```python
from build123d import *

# Parameters (mm, degrees)
SKETCH1_W               = 82.8
SKETCH1_H               = 213.8
SKETCH1_R               = 0.8
PCB_EXTRUDE_DEPTH       = 1.6
SKETCH3_R               = 1.5
SOLAR_HOLE_DEPTH        = 1.6
CUT_EXTRUDE1_DEPTH      = 115.647852139
CUT_EXTRUDE1_DEPTH_BACK = 115.647852139
SKETCH8_W               = 82.8
SKETCH8_H               = 114.4
M2_CLEARANCE_HOLE1_D    = 2.6


with BuildPart() as part:
    # Sketch1 → pcb extrude (new body)
    with BuildSketch(Plane.XY):
        Rectangle(SKETCH1_W, SKETCH1_H)
        with Locations((-39.5, -27)):
            Circle(SKETCH1_R, mode=Mode.SUBTRACT)
        with Locations((39.5, -27)):
            Circle(SKETCH1_R, mode=Mode.SUBTRACT)
        with Locations((-39.5, 87)):
            Circle(SKETCH1_R, mode=Mode.SUBTRACT)
        with Locations((-39.5, 57)):
            Circle(SKETCH1_R, mode=Mode.SUBTRACT)
        with Locations((-39.5, 27)):
            Circle(SKETCH1_R, mode=Mode.SUBTRACT)
        with Locations((-39.5, -57)):
            Circle(SKETCH1_R, mode=Mode.SUBTRACT)
        with Locations((-39.5, -87)):
            Circle(SKETCH1_R, mode=Mode.SUBTRACT)
        with Locations((0, -104.2)):
            Circle(SKETCH1_R, mode=Mode.SUBTRACT)
        with Locations((39.5, -87)):
            Circle(SKETCH1_R, mode=Mode.SUBTRACT)
        with Locations((39.5, -57)):
            Circle(SKETCH1_R, mode=Mode.SUBTRACT)
        with Locations((39.5, 27)):
            Circle(SKETCH1_R, mode=Mode.SUBTRACT)
        with Locations((39.5, 57)):
            Circle(SKETCH1_R, mode=Mode.SUBTRACT)
        with Locations((39.5, 87)):
            Circle(SKETCH1_R, mode=Mode.SUBTRACT)
        with Locations((0, 104.2)):
            Circle(SKETCH1_R, mode=Mode.SUBTRACT)
    extrude(amount=PCB_EXTRUDE_DEPTH)

    # Sketch3 → Solar Hole (cut)
    with BuildSketch(Plane.XY.offset(1.6)):
        with Locations((0, 104.2)):
            Circle(SKETCH3_R)
        with BuildLine():
            Line((-2.5, 101.4), (2.5, 101.4))
            Line((2.5, 101.4), (2.5, 104.9))
            Line((2.5, 104.9), (9.5, 104.9))
            ThreePointArc((9.5, 104.9), (10, 104.4), (9.5, 103.9))
            Line((9.5, 103.9), (6.2, 103.9))
            Line((6.2, 103.9), (6.2, 101.4))
            Line((6.2, 101.4), (6.2, 96.6))
            Line((6.2, 96.6), (-6.2, 96.6))
            Line((-6.2, 96.6), (-6.2, 101.4))
            Line((-6.2, 101.4), (-6.2, 103.9))
            Line((-6.2, 103.9), (-9.5, 103.9))
            ThreePointArc((-9.5, 103.9), (-10, 104.4), (-9.5, 104.9))
            Line((-9.5, 104.9), (-2.5, 104.9))
            Line((-2.5, 104.9), (-2.5, 101.4))
        make_face()
    extrude(amount=-SOLAR_HOLE_DEPTH, mode=Mode.SUBTRACT)

    # Sketch8 → Cut-Extrude1 (cut, two sides: drawn at the far end of the back side and taken through both)
    with BuildSketch(Plane.XY.offset(1.6).offset(-CUT_EXTRUDE1_DEPTH_BACK)):
        with Locations((0, -49.7)):
            Rectangle(SKETCH8_W, SKETCH8_H)
    extrude(amount=CUT_EXTRUDE1_DEPTH + CUT_EXTRUDE1_DEPTH_BACK, mode=Mode.SUBTRACT)

    # M2 Clearance Hole1 (through all)
    with Locations(Plane(origin=(0, 0, 0), x_dir=(-1, 0, 0), z_dir=(0, 0, -1))):
        with Locations((39.5, 87), (-39.5, 87), (39.5, 57), (-39.5, 57), (39.5, 27), (-39.5, 27), (16.5, 77.25), (-16.5, 77.25), (-16.5, 37.25), (16.5, 37.25)):
            Hole(M2_CLEARANCE_HOLE1_D / 2)


solid = part.part
```
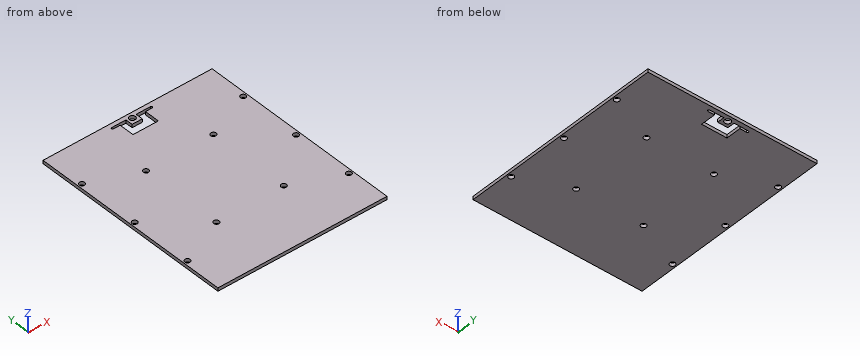
Geometry: final body of the model. Coordinates: model frame, mm. Round coordinates to 2 decimals unless told otherwise and drop trailing zeros. Order: outer loops, then holes, each group sorted by start corner. A loop starts at its lowest first (then second) coordinate and runs counter-clockwise, first axis right, second up. Notation, with made-up numbers: (65, -4) - (90, -4) arc R20 ccw to (90, 6) - close; hole circle Ø6 at (-12.75, -19). An arc over 180 degrees is marked (long way). Write item = value, one per line. Start each with the question number.
Q1. Pin query (flat end, axial travel): pin 1 (1.6 mm diameter, centred on x = 16.5, y = 37.25, fed in from +Z). Return the tip coordinate at first contact, or that it passes through.
Q2. Cut plane D-D on x = 4. Return the cut outline in (y, z).
Q3. Cut plane B-B on y = 87. Return the cut outline in (x, z).
Q4. Ray query, line 1 (Y direction, x = 39.5, z = 1.25); line 2 (Y direction, x = 16.5, z = 0.6); line 3 (Y direction, x = 0, z = 0.55). Return the intervals inside material, ascending. Write a range as from..to.
Q5. Cut plane A-A on x = 39.5. Return the cut outline in (y, z).
Q6. Cut plane C-C on z = 1.25. Give the number of separate pieces and of enclosed holes in the cut face, and give its area (3 significant figures).
Outcome:
q1.pin_1 = through
q2.outline = (7.5, 0) - (96.6, 0) - (96.6, 1.6) - (7.5, 1.6) - close; (104.9, 0) - (106.9, 0) - (106.9, 1.6) - (104.9, 1.6) - close
q3.outline = (-41.4, 0) - (-40.8, 0) - (-40.8, 1.6) - (-41.4, 1.6) - close; (-38.2, 0) - (38.2, 0) - (38.2, 1.6) - (-38.2, 1.6) - close; (40.8, 0) - (41.4, 0) - (41.4, 1.6) - (40.8, 1.6) - close
q4.line_1 = 7.5..25.7, 28.3..55.7, 58.3..85.7, 88.3..106.9
q4.line_2 = 7.5..35.95, 38.55..75.95, 78.55..106.9
q4.line_3 = 7.5..96.6, 101.4..102.7, 105.7..106.9
q5.outline = (7.5, 0) - (25.7, 0) - (25.7, 1.6) - (7.5, 1.6) - close; (28.3, 0) - (55.7, 0) - (55.7, 1.6) - (28.3, 1.6) - close; (58.3, 0) - (85.7, 0) - (85.7, 1.6) - (58.3, 1.6) - close; (88.3, 0) - (106.9, 0) - (106.9, 1.6) - (88.3, 1.6) - close
q6.separate_pieces = 1
q6.enclosed_holes = 12
q6.area = 8,080 mm^2
